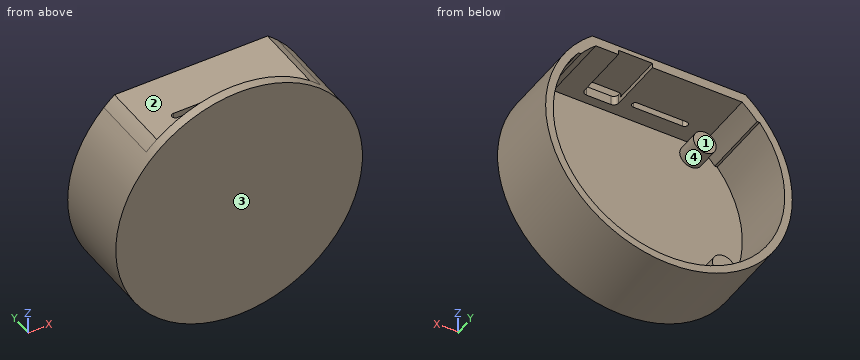
```python
from build123d import *
from build123d.topology import SkipClean

# Parameters (mm, degrees)
SKETCH1_R           = 32.5
BOSS_EXTRUDE1_DEPTH = 21
SHELL1_T            = -2.5
CUT_EXTRUDE2_START  = -18.5
CUT_EXTRUDE2_DEPTH  = 18.5
BOSS_EXTRUDE2_DEPTH = 18.5
CUT_EXTRUDE4_DEPTH  = 18.5
SKETCH9_R           = 3
BOSS_EXTRUDE3_DEPTH = 6
CUT_EXTRUDE3_REACH  = 71.707
SKETCH8_W           = 8.98
SKETCH8_H           = 14.74
CUT_EXTRUDE5_DEPTH  = 1.25


with BuildPart() as part:
    # Sketch1 → Boss-Extrude1 (new body)
    with BuildSketch(Plane(origin=(0, 0, 0), x_dir=(1, 0, 0), z_dir=(0, 1, 0))):
        with Locations(Location((0, 0, 0), (0, 0, 90))):
            Circle(SKETCH1_R)
    extrude(amount=BOSS_EXTRUDE1_DEPTH)

    # Shell1
    shell1_openings = [part.faces().sort_by_distance(p)[0] for p in [
        (0, 21, 0),
    ]]
    offset(amount=SHELL1_T, openings=shell1_openings, kind=Kind.INTERSECTION)

    # Sketch4 → Cut-Extrude2 (cut)
    with BuildSketch(Plane(origin=(0, 21, 0), x_dir=(1, 0, 0), z_dir=(0, 1, 0)).offset(CUT_EXTRUDE2_START)):
        with BuildLine():
            Line((-19.2835, -22.981440942), (19.2835, -22.981440942))
            Line((19.2835, -22.981440942), (22.980499826, -22.981440942))
            ThreePointArc((22.980499826, -22.981440942), (0, -32.5), (-22.980499826, -22.981440942))
            Line((-22.980499826, -22.981440942), (-19.2835, -22.981440942))
        make_face()
    extrude(amount=CUT_EXTRUDE2_DEPTH, mode=Mode.SUBTRACT)

    # Sketch5 → Boss-Extrude2 (add, through all)
    with SkipClean():  # the faces are left unmerged after this step: merging them gives an invalid solid
        with BuildSketch(Plane(origin=(0, 2.5, 0), x_dir=(1, 0, 0), z_dir=(0, 1, 0))):
            with BuildLine():
                Line((-22.980499826, -22.981440942), (22.980499826, -22.981440942))
                ThreePointArc((22.980499826, -22.981440942), (21.612881002, -24.27206985), (20.17290677, -25.481440942))
                Line((20.17290677, -25.481440942), (-20.17290677, -25.481440942))
                ThreePointArc((-20.17290677, -25.481440942), (-21.612881002, -24.27206985), (-22.980499826, -22.981440942))
            make_face()
        extrude(amount=BOSS_EXTRUDE2_DEPTH)

    # Sketch7 → Cut-Extrude4 (cut)
    with SkipClean():  # the faces are left unmerged after this step: merging them gives an invalid solid
        with BuildSketch(Plane(origin=(0, 21, 0), x_dir=(1, 0, 0), z_dir=(0, 1, 0))):
            with BuildLine():
                Line((-23.231549664, -18.981440942), (-23.873728234, -18.981440942))
                ThreePointArc((-23.873728234, -18.981440942), (0, 30.5), (23.873728234, -18.981440942))
                Line((23.873728234, -18.981440942), (23.231549664, -18.981440942))
                Line((23.231549664, -18.981440942), (-23.231549664, -18.981440942))
            make_face()
        extrude(amount=-CUT_EXTRUDE4_DEPTH, mode=Mode.SUBTRACT)

    # Sketch9 → Boss-Extrude3 (add)
    with SkipClean():  # the faces are left unmerged after this step: merging them gives an invalid solid
        with BuildSketch(Plane(origin=(0, 2.5, 0), x_dir=(1, 0, 0), z_dir=(0, 1, 0))):
            with Locations(Location((-22, 15, 0), (0, 0, 270))):
                Circle(SKETCH9_R)
            with Locations(Location((22, 15, 0), (0, 0, 270))):
                Circle(SKETCH9_R)
            with Locations(Location((-17, -19, 0), (0, 0, 270))):
                Circle(SKETCH9_R)
        extrude(amount=BOSS_EXTRUDE3_DEPTH)

    # Sketch6 → Cut-Extrude3 (cut, up to next)
    with BuildSketch(Plane.XY.offset(25.481440942), mode=Mode.PRIVATE) as cut_extrude3_sk1:
        with BuildLine():
            Line((-12.2, 8.5), (0.8, 8.5))
            ThreePointArc((0.8, 8.5), (1.667712103, 7.632287897), (0.8, 6.764575794))
            Line((0.8, 6.764575794), (-12.2, 6.764575794))
            ThreePointArc((-12.2, 6.764575794), (-13.067712103, 7.632287897), (-12.2, 8.5))
        make_face()
    cut_extrude3_tool1 = extrude(cut_extrude3_sk1.sketch, amount=-CUT_EXTRUDE3_REACH, mode=Mode.PRIVATE) & part.part
    # Sketch6 → Cut-Extrude3 (cut, up to next)
    with BuildSketch(Plane.XY.offset(25.481440942), mode=Mode.PRIVATE) as cut_extrude3_sk2:
        with BuildLine():
            Line((5.64, 4.97), (12.04, 4.97))
            ThreePointArc((12.04, 4.97), (12.952167748, 5.347832252), (13.33, 6.26))
            Line((13.33, 6.26), (13.33, 6.98))
            ThreePointArc((13.33, 6.98), (12.952167748, 7.892167748), (12.04, 8.27))
            Line((12.04, 8.27), (5.64, 8.27))
            ThreePointArc((5.64, 8.27), (4.727832252, 7.892167748), (4.35, 6.98))
            Line((4.35, 6.98), (4.35, 6.26))
            ThreePointArc((4.35, 6.26), (4.727832252, 5.347832252), (5.64, 4.97))
        make_face()
    cut_extrude3_tool2 = extrude(cut_extrude3_sk2.sketch, amount=-CUT_EXTRUDE3_REACH, mode=Mode.PRIVATE) & part.part
    add(cut_extrude3_tool1.solids().sort_by_distance((-5.7, 7.632288, 25.481441))[0], mode=Mode.SUBTRACT)
    add(cut_extrude3_tool2.solids().sort_by_distance((8.84, 6.62, 25.481441))[0], mode=Mode.SUBTRACT)

    # Sketch8 → Cut-Extrude5 (cut)
    with SkipClean():  # the faces are left unmerged after this step: merging them gives an invalid solid
        with BuildSketch(Plane(origin=(0, 0, 22.981440942), x_dir=(-1, 0, 0), z_dir=(0, 0, -1))):
            with Locations((-8.84, 13.63)):
                Rectangle(SKETCH8_W, SKETCH8_H)
        extrude(amount=-CUT_EXTRUDE5_DEPTH, mode=Mode.SUBTRACT)


solid = part.part
```
Geometry: final body of the model. Coordinates: model frame, mm. Face numbers are marked on the shaded views. A direction names the side the tool comes from. Round coordinates to 2 decimals unless told otherwise and drop trailing zeros. Write each loop counter-clockwise with the first axis right and the second up, starting at its lowest first coordinate (ties: lowest second). Pieces come first, ordered by that corner, then holes. Notation, with made-up numbers: M 70,85.5 L 87,85.5 A25 ccw 87,118.5 Z; hole C 38,-4 d6. An arc over 180 degrees is marked long. Answer in a Markdown table with one row per item. Add a question column.
(1) Cut plane B-B, the plane y = 12.5. Return the cut outline in (x, z), then the cut area to 3 significant figures.
(2) Contact query for flat-ended pins moving along their axis: pin 1 (9 mm diameter, centred on x = -5.5, y = 10, fed in from -Z); pin 2 (2 mm diameter, centred on y = 13, z = 24.5, fed in from -X); pin 3 (6 mm diameter, centred on y = 19, z = 13, fed in from +X). Output: stop coordinate, or through.
(3) Ray query, L1, parallel to X at y = 16.25, z = 0; L2, parallel to Y at x = -5, z = 23.5; L3, parallel to Z at x = -24, y = 4.75. Return the intervals inside material, ascending.
(4) Cut plane C-C, the plane z = 0. Return the cut outline in (x, y), then the cut area to 4 significant figures.
(5) Draft query along X for the marked faces 1 and 2. Return one class per face: pulls with the +X half, pulls with the -X half, needs draft (parallel to the pull), parting line crosses it, or undercut.
(6) Reachability of the marked faces 3 and 4 from +Z, -Z, +X, -X, +Y, -Y: full face, straight path, thin tool, end or side. Return the list, or none.
(7) Cut plane D-D, the plane x = -22. Return the cut outline in (y, z).
(8) Cut plane A-A, the plane x = 0. Return the cut outline in (y, z), then the cut area to 3 significant figures.
Established:
| question | item | result |
|---|---|---|
| 1 | outline | M -20.17,25.48 A32.5 ccw long 20.17,25.48 Z; hole M -23.87,18.98 A30.5 ccw long 23.87,18.98 L 23.23,18.98 A30 ccw 19.28,22.98 L 13.33,22.98 L 13.33,24.23 L 4.35,24.23 L 4.35,22.98 L -19.28,22.98 A30 ccw -23.23,18.98 Z |
| 1 | area | 403 mm² |
| 2 | pin 1 | z = -32.48 |
| 2 | pin 2 | x = -22.45 |
| 2 | pin 3 | x = 30.92 |
| 3 | L1 | -32.5 to -30.5, 30.5 to 32.5 |
| 3 | L2 | 0 to 6.76, 8.5 to 21 |
| 3 | L3 | -21.91 to -18.82, -17.24 to -12.76, 18.82 to 21.91 |
| 4 | outline | M -32.5,0 L 32.5,0 L 32.5,21 L 30.5,21 L 30.5,2.5 L -30.5,2.5 L -30.5,21 L -32.5,21 Z |
| 4 | area | 236.5 mm² |
| 5 | face 1 | undercut |
| 5 | face 2 | needs draft |
| 6 | face 3 | +Z, -Z, +X, -X, -Y |
| 6 | face 4 | +Y |
| 7 | outline | M 0,-23.92 L 21,-23.92 L 21,-21.12 L 2.5,-21.12 L 2.5,-18 L 8.5,-18 L 8.5,-12 L 2.5,-12 L 2.5,20.4 L 21,20.4 L 21,23.92 L 0,23.92 Z |
| 8 | outline | M 0,-32.5 L 21,-32.5 L 21,-30.5 L 2.5,-30.5 L 2.5,22.98 L 6.76,22.98 L 6.76,25.48 L 2.5,25.48 L 2.5,32.5 L 0,32.5 Z; M 8.5,22.98 L 21,22.98 L 21,25.48 L 8.5,25.48 Z |
| 8 | area | 241 mm² |
